Design review of the part shown in the three views and the two pictorial views. Dimensions are in mm from the part's minimum x, y and z. A direction names the side the tool comes from. Give positions to 0.01 mm unless a question says otherwise; leave off trailing zeros. Order: outer loops, then holes, each group sorted by start corner. A loop starts at its lowest first (then second) coordinate and runs counter-clockwise, first axis right, second up. Notation, with made-up numbers: (-12, 33) - (28, 33) arc R22 cw to (28, 43) - close; hole circle Ø4 at (80.5, 70.5). An arc over 180 degrees is marked (long way). Put each result on its own line as item: value.
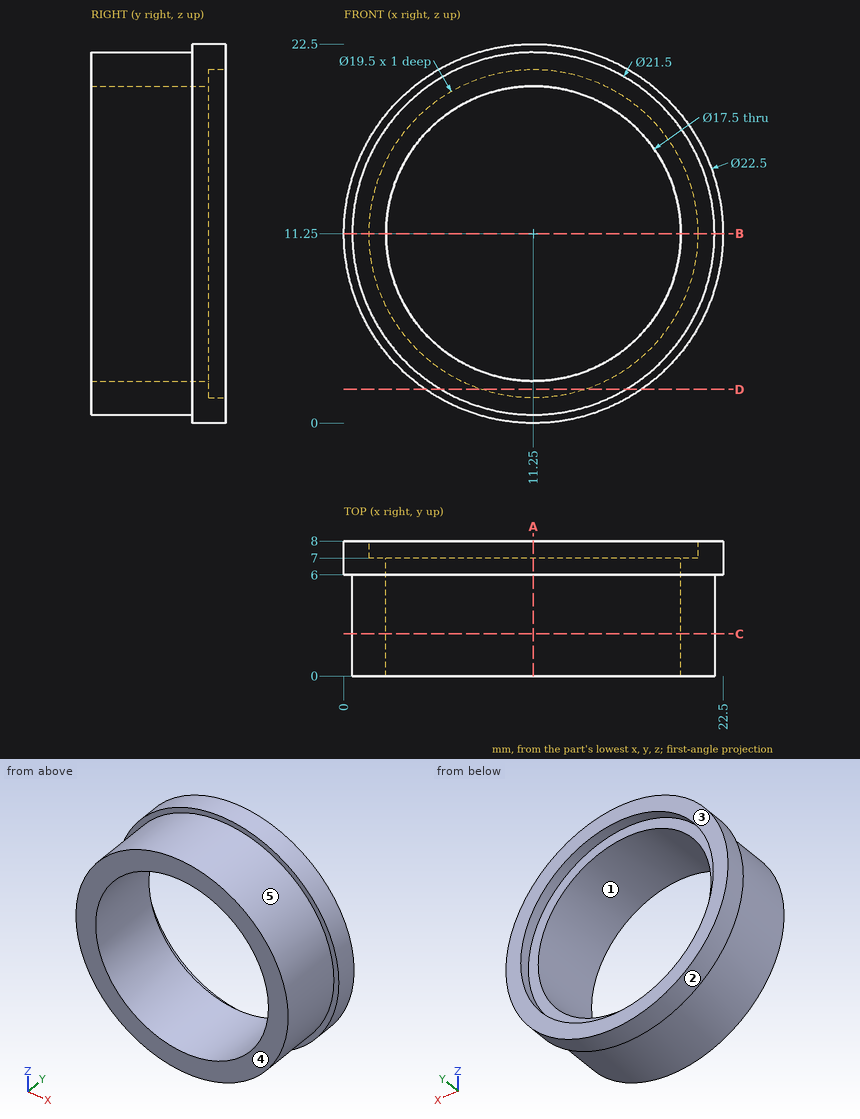
(1) Take a section at B-B, the plane z = 11.25. Write out the cut boundary in (x, y), then the cut area to 3 significant figures.
The answers:
outline: (0, 6) - (0.5, 6) - (0.5, 0) - (2.5, 0) - (2.5, 7) - (1.5, 7) - (1.5, 8) - (0, 8) - close; (20, 0) - (22, 0) - (22, 6) - (22.5, 6) - (22.5, 8) - (21, 8) - (21, 7) - (20, 7) - close
area: 32.0 mm^2
(2) Clearance check with flat-ended pins moving along their axes: pin 1 Ø1 at (y, z) = (1.5, 3) entering from +X; pin 2 Ø3 at (x, y) = (3, 6.5) entering from -Z. State where each tip first meets the part, or that it passes through.
The answers:
pin 1: x = 18.7
pin 2: z = 2.25
(3) For the marked faces 4 and 5, list the 3-axis set-ups (+Z, -Z, +X, -X, +Y, -Y) from which the entire face can be reached by the end or side of a thin tool; tool diameter is ignored.
The answers:
face 4: +Z, -Z, +X, -X, -Y
face 5: -Y
(4) The part is to be moulded in two halves that separate along X. For the marked faces 1, 2 and 3, say which applies: pulls with the +X half, pulls with the -X half, needs draft (parallel to the pull), parting line crosses it, or undercut.
The answers:
face 1: undercut
face 2: parting line crosses it
face 3: needs draft
(5) Take a section at C-C, the plane y = 2.5. Write out the cut boundary in (x, z).
The answers:
outline: circle Ø21.5 at (11.25, 11.25); hole circle Ø17.5 at (11.25, 11.25)
(6) Take a section at D-D, the plane z = 2. Write out the cut boundary in (x, y).
The answers:
outline: (4.85, 6) - (5.77, 6) - (5.77, 0) - (16.73, 0) - (16.73, 6) - (17.65, 6) - (17.65, 8) - (14.33, 8) - (14.33, 7) - (8.17, 7) - (8.17, 8) - (4.85, 8) - close
(7) Wall thickness on L1, parallel to Z at x = 11.25, y = 7.75; L2, parallel to Z at x = 11.25, y = 1.5; L3, parallel to X at y = 5.5, z = 15.25: over which ranges is each line inside the solid? List them lowest first.
The answers:
L1: 0 to 1.5, 21 to 22.5
L2: 0.5 to 2.5, 20 to 22
L3: 1.27 to 3.47, 19.03 to 21.23
(8) Take a section at A-A, the plane x = 11.25. Write out the cut boundary in (y, z).
The answers:
outline: (0, 0.5) - (6, 0.5) - (6, 0) - (8, 0) - (8, 1.5) - (7, 1.5) - (7, 2.5) - (0, 2.5) - close; (0, 20) - (7, 20) - (7, 21) - (8, 21) - (8, 22.5) - (6, 22.5) - (6, 22) - (0, 22) - close
